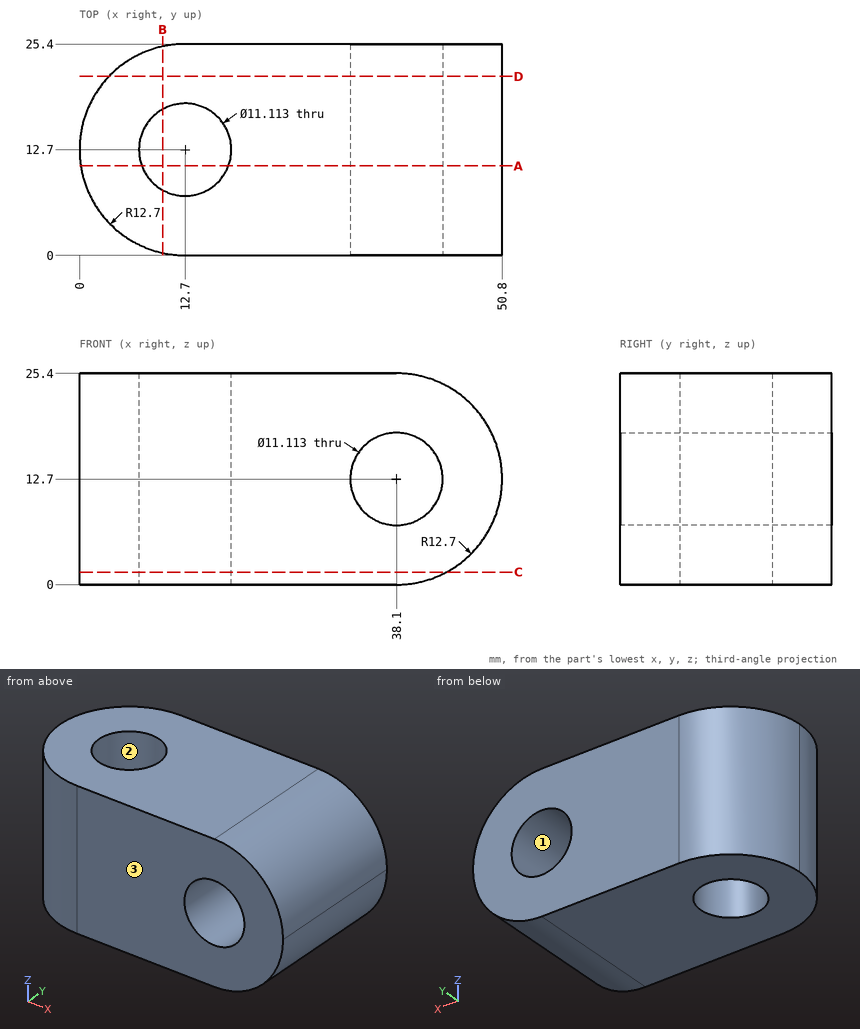
Check sheet for the drawn part. Datum: minimum x, y, z corner. Units: mm. Coordinates: 2 decimals unless noted, no trailing zeros. Loops run counter-clockwise (first coordinate to the right, second up) from the corner with the lowest first, then second, coordinate; pieces in that order, holes last. Notation, with made-up numbers: (12.5, 22.5) -> (29.5, 22.5) arc R11 ccw to (29.5, 41.5) -> close; hole circle Ø7 at (24.5, 47). An arc over 180 degrees is marked (long way). Answer as a JSON object with one key per item and string values. Group by question number.
Item 1: Sectioned sample at A-A on y = 10.75. Record the boundary of the cut face in (x, z).
Item 2: Scan lines: probe 1 along Y at (x, z) = (13, 23.75); probe 2 along Z at (x, y) = (38.1, 16.25); probe 3 along X at (y, z) = (11, 12.7) (1 decimal). Record each from-to range of solid material in increasing order.
Item 3: Mould release check, pull along Y, two halves, no side actions. Record for the marked faces 1, 2 and 3: +Y half, -Y half, draft (parallel to the pull), parting line (faces both ways), or undercut.
Item 4: Sectioned sample at D-D on y = 21.5. Record the boundary of the cut face in (x, z), plus the area to 3 significant figures.
Item 5: Sectioned sample at B-B on x = 10. Record the boundary of the cut face in (y, z), plus the area to 3 significant figures.
Item 6: Sectioned sample at C-C on z = 1.5. Record the boundary of the cut face in (x, y).
Item 7: Depth check by flat-ended pin: pin 1 (8 mm diameter, centred on y = 9.5, z = 20.5, fed in from -X); pin 2 (10 mm diameter, centred on x = 12.7, y = 12.7, fed in from +Z); pin 3 (1 mm diameter, centred on x = 39.5, y = 5.5, fed in from -Z); pin 4 (1 mm diameter, centred on y = 11, z = 13, fed in from -X). Enter the tip coordinate at first touch or a pass-through.
Evaluation:
{
 "1": {"outline": "(0.15, 0) -> (7.5, 0) -> (7.5, 25.4) -> (0.15, 25.4) -> close; (17.9, 0) -> (38.1, 0) arc R12.7 ccw to (38.1, 25.4) -> (17.9, 25.4) -> close; hole circle Ø11.11 at (38.1, 12.7)"},
 "2": {"probe 1": "y = 0 to 7.15, 18.25 to 25.4", "probe 2": "z = 0 to 7.14, 18.26 to 25.4", "probe 3": "x = 0.1 to 7.4, 18 to 32.5, 43.7 to 50.8"},
 "3": {"face 1": "draft", "face 2": "undercut", "face 3": "-Y half"},
 "4": {"outline": "(3.54, 0) -> (38.1, 0) arc R12.7 ccw to (38.1, 25.4) -> (3.54, 25.4) -> close; hole circle Ø11.11 at (38.1, 12.7)", "area": "1,030 mm²"},
 "5": {"outline": "(0.29, 0) -> (7.84, 0) -> (7.84, 25.4) -> (0.29, 25.4) -> close; (17.56, 0) -> (25.11, 0) -> (25.11, 25.4) -> (17.56, 25.4) -> close", "area": "384 mm²"},
 "6": {"outline": "(12.7, 0) -> (44.09, 0) -> (44.09, 25.4) -> (12.7, 25.4) arc R12.7 ccw to start; hole circle Ø11.11 at (12.7, 12.7)"},
 "7": {"pin 1": "stops at x = 0", "pin 2": "passes through", "pin 3": "stops at z = 0.03", "pin 4": "stops at x = 0.06"}
}
